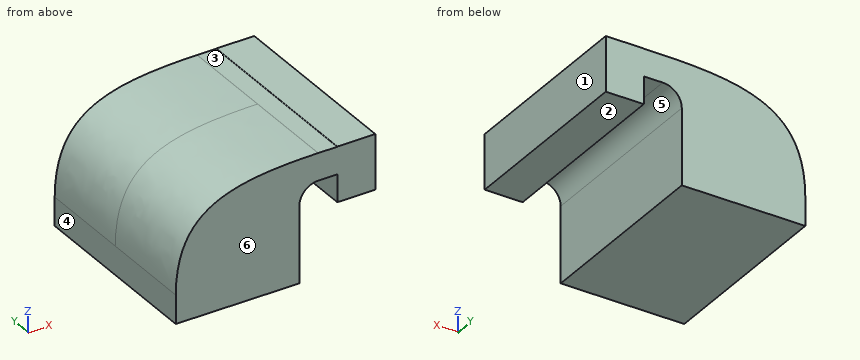
```python
from build123d import *

# Parameters (mm, degrees)
F1_DEPTH = 63.5


with BuildPart() as f1:
    # F0 (on Front) → F1 (new body, symmetric)
    with BuildSketch(Plane.XZ):
        Polygon((-41.275, -9.525), (41.275, -9.525), (41.275, 9.525), (23.111848, 9.525), (-41.275, 9.525), align=None)
        with BuildLine():
            Line((23.111848, 9.525), (41.275, 9.525))
            Line((41.275, 9.525), (41.275, 41.275))
            ThreePointArc((41.275, 41.275), (44.994744, 50.255256), (53.975, 53.975))
            Line((53.975, 53.975), (66.675, 53.975))
            Line((66.675, 53.975), (66.675, 72.138152))
            Line((66.675, 72.138152), (53.975, 72.138152))
            ThreePointArc((53.975, 72.138152), (53.883431, 72.138016), (53.791864, 72.137608))
            ThreePointArc((53.791864, 72.137608), (32.086803, 63.033699), (23.111848, 41.275))
            Line((23.111848, 41.275), (23.111848, 9.525))
        make_face()
        with BuildLine():
            add(Edge.make_bspline(
                [(-41.275, 9.525), (-40.953308, 63.672334), (-6.200092, 71.951322), (53.791864, 72.137608)],
                knots=[0, 0, 0, 0, 113.870886, 113.870886, 113.870886, 113.870886], degree=3))
            Line((-41.275, 9.525), (23.111848, 9.525))
            Line((23.111848, 9.525), (23.111848, 41.275))
            ThreePointArc((23.111848, 41.275), (32.086803, 63.033699), (53.791864, 72.137608))
        make_face()
        Polygon((66.675, 72.138152), (66.675, 53.975), (66.675, 35.663907), (92.075, 35.663907), (92.075, 72.286093), (66.675, 72.286093), align=None)
    extrude(amount=F1_DEPTH, both=True)


solid = f1.part
```
Here's how the part is built. I have some questions about the finished solid (model axes, mm). Face numbers are marked on the shaded views. A direction names the side the tool comes from. Round coordinates to 2 decimals unless told otherwise and drop trailing zeros. Write each loop counter-clockwise with the first axis right and the second up, starting at its lowest first coordinate (ties: lowest second). Pieces come first, ordered by that corner, then holes.
Q1. Please list where these lines run through material, in increasing order: probe 1 along Z at (x, y) = (78, -10); probe 2 along X at (y, z) = (4.5, 46.5) (3 decimals); probe 3 along X at (y, z) = (10.5, 41) (3 decimals).
Q2. Which directions (+Z, -Z, +X, -X, +Y, -Y) give clear straight access to the entire face, cutting with the end or side of a thin tool? Please do the marked faces 1, 2 and 3.
Q3. If we section it at A-A on x = 64: Write out the boundary of the cut face in (y, z) (3 decimals).
Q4. Will these pins go through, and if not, where does the flat tip stop? P1, Ø6.5, axis at x = 63, y = 24, coming from the -Z side (3 decimals); P2, Ø6, axis at y = -24.5, z = 6.5, coming from the +X side (3 decimals); P3, Ø6.5, axis at x = 58.5, y = 25, coming from the +Z side.
Q5. If we section it at B-B on z = -3: Write out the boundary of the cut face in (x, y) (3 decimals), plus the area to 3 significant figures.
Q6. If we mould it in two halves opening along X, with no side actions, what happens to the marked faces 4, 5 and 6? For each: +X half, -X half, draft (parallel to the pull), parting line (faces both ways), or undercut.
Answer below:
1. probe 1: z = 35.66 to 72.29
1. probe 2: x = -32.198 to 42.4, 66.675 to 92.075
1. probe 3: x = -35.272 to 41.275, 66.675 to 92.075
2. face 1: +Z, -Z, +X, +Y, -Y
2. face 2: -Z, +X, +Y, -Y
2. face 3: +Z, -X, +Y, -Y
3. outline: (-63.5, 53.975) - (63.5, 53.975) - (63.5, 72.138) - (-63.5, 72.138) - close
4. P1: stops at z = 53.975
4. P2: stops at x = 41.275
4. P3: stops at z = 72.14
5. outline: (-41.275, -63.5) - (41.275, -63.5) - (41.275, 63.5) - (-41.275, 63.5) - close
5. area: 10,500 mm2
6. face 4: -X half
6. face 5: undercut
6. face 6: draft
